CAD build for the part. Positions are in the model's coordinates, mm. Face numbers are marked on the shaded views. A direction names the side the tool comes from. Round coordinates to 2 decimals unless told otherwise and drop trailing zeros. Loops run counter-clockwise (first coordinate to the right, second up) from the corner with the lowest first, then second, coordinate; pieces in that order, holes last. Notation, with made-up numbers: (16.5, 37.5) - (46.5, 37.5) arc R21 cw to (46.5, 67.5) - close; hole circle Ø10 at (80.25, -12). An arc over 180 degrees is marked (long way). Use one line per item in the form item = value.
from build123d import *

# Parameters (mm, degrees)
SALIENTE_EXTRUIR1_DEPTH = 30
CROQUIS2_R              = 0.8
CORTAR_EXTRUIR1_DEPTH   = 2
CROQUIS3_R              = 0.85
CORTAR_EXTRUIR2_DEPTH   = 2
CORTAR_EXTRUIR3_DEPTH   = 2


with BuildPart() as part:
    # Croquis1 → Saliente-Extruir1 (new body)
    with BuildSketch(Plane.XY):
        Polygon((0, 0), (0, 81), (2, 81), (2, 2), (50, 2), (50, 38.5), (52, 38.5), (52, 0), align=None)
    extrude(amount=SALIENTE_EXTRUIR1_DEPTH)

    # Croquis2 → Cortar-Extruir1 (cut)
    with BuildSketch(Plane(origin=(52, 0, 0), x_dir=(0, 0, -1), z_dir=(1, 0, 0))):
        with Locations(Location((-25.3, 33.8, 0), (0, 0, 90))):
            Circle(CROQUIS2_R)
    extrude(amount=-CORTAR_EXTRUIR1_DEPTH, mode=Mode.SUBTRACT)

    # Croquis3 → Cortar-Extruir2 (cut)
    with BuildSketch(Plane.ZY):
        with Locations((4.55, 77.25)):
            Circle(CROQUIS3_R)
        with Locations((25.45, 77.25)):
            Circle(CROQUIS3_R)
        with Locations((25.45, 51.45)):
            Circle(CROQUIS3_R)
        with Locations((4.55, 51.45)):
            Circle(CROQUIS3_R)
        with Locations(Location((25.45, 29.55, 0), (0, 0, 270))):
            Circle(CROQUIS3_R)
        with Locations(Location((4.55, 29.55, 0), (0, 0, 270))):
            Circle(CROQUIS3_R)
        with Locations(Location((25.45, 3.75, 0), (0, 0, 270))):
            Circle(CROQUIS3_R)
        with Locations(Location((4.55, 3.75, 0), (0, 0, 270))):
            Circle(CROQUIS3_R)
        with Locations((8.7, 40.5)):
            Circle(CROQUIS3_R)
        with Locations((21.3, 40.5)):
            Circle(CROQUIS3_R)
    extrude(amount=-CORTAR_EXTRUIR2_DEPTH, mode=Mode.SUBTRACT)

    # Croquis4 → Cortar-Extruir3 (cut)
    with BuildSketch(Plane.XZ):
        with BuildLine():
            Line((4.95, 25.4), (8.55, 25.4))
            ThreePointArc((8.55, 25.4), (10.4, 23.55), (8.55, 21.7))
            Line((8.55, 21.7), (4.95, 21.7))
            ThreePointArc((4.95, 21.7), (3.1, 23.55), (4.95, 25.4))
        make_face()
        with BuildLine():
            Line((42.55, 25.4), (46.15, 25.4))
            ThreePointArc((46.15, 25.4), (48, 23.55), (46.15, 21.7))
            Line((46.15, 21.7), (42.55, 21.7))
            ThreePointArc((42.55, 21.7), (40.7, 23.55), (42.55, 25.4))
        make_face()
        with BuildLine():
            Line((18, 23.55), (18, 30))
            ThreePointArc((18, 30), (21.5, 33.5), (25, 30))
            Line((25, 30), (25, 23.55))
            ThreePointArc((25, 23.55), (21.5, 20.05), (18, 23.55))
        make_face()
    extrude(amount=-CORTAR_EXTRUIR3_DEPTH, mode=Mode.SUBTRACT)


solid = part.part
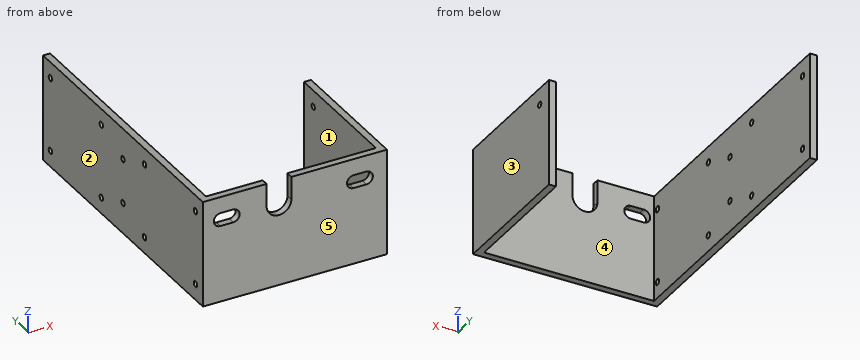
1) Slice it at D-D (x = 13.5). Write the cut outline in (y, z), plus the area to 3 significant figures.
Report:
outline = (0, 0) - (2, 0) - (2, 30) - (0, 30) - close
area = 60.0 mm^2
2) Slice it at C-C (z = 15.75). Write the cut outline in (x, y).
Report:
outline = (0, 0) - (52, 0) - (52, 38.5) - (50, 38.5) - (50, 2) - (2, 2) - (2, 81) - (0, 81) - close
3) Two-plate mould, pull along X, no slides. Class the marked faces 1, 2 and 3: +X half, -X half, draft (parallel to the pull), parting line (faces both ways), or undercut.
Report:
face_1 = undercut
face_2 = -X half
face_3 = +X half
4) Flat gauge pins, fed straight in: pin 1 (15 mm diameter, centred on y = 48.5, z = 10.5, fed in from +X); pin 2 (6 mm diameter, centred on x = 41, z = 26, fed in from -Y); pin 3 (1.6 mm diameter, centred on x = 50.5, z = 12.5, fed in from +Y). Where does each tip first touch, or does it go through?
Report:
pin_1 = 2
pin_2 = 0
pin_3 = 38.5
5) Drill centre lines: probe 1 along Z at (x, y) = (0.55, 3.75); probe 2 along X at (y, z) = (32, 25); probe 3 along Y at (x, z) = (13.5, 6.75). Where is each one in solid material? Low to high.
Report:
probe_1 = 0 to 3.7, 5.4 to 24.6, 26.3 to 30
probe_2 = 0 to 2, 50 to 52
probe_3 = 0 to 2
6) Tool access for the marked faces 4 and 5: list every direction of +Z, -Z, +X, -X, +Y, -Y with a clear straight run to the whole face (end or side of a thin tool).
Report:
face_4 = +Z, -Z, +Y
face_5 = +Z, -Z, +X, -X, -Y
7) Slice it at B-B (y = 77.25). Write the cut outline in (x, z), plus the area to 3 significant figures.
Report:
outline = (0, 0) - (2, 0) - (2, 3.7) - (0, 3.7) - close; (0, 5.4) - (2, 5.4) - (2, 24.6) - (0, 24.6) - close; (0, 26.3) - (2, 26.3) - (2, 30) - (0, 30) - close
area = 53.2 mm^2
8) Slice it at A-A (y = 3.75). Write the cut outline in (x, z).
Report:
outline = (0, 0) - (2, 0) - (2, 3.7) - (0, 3.7) - close; (0, 5.4) - (2, 5.4) - (2, 24.6) - (0, 24.6) - close; (0, 26.3) - (2, 26.3) - (2, 30) - (0, 30) - close; (50, 0) - (52, 0) - (52, 30) - (50, 30) - close
